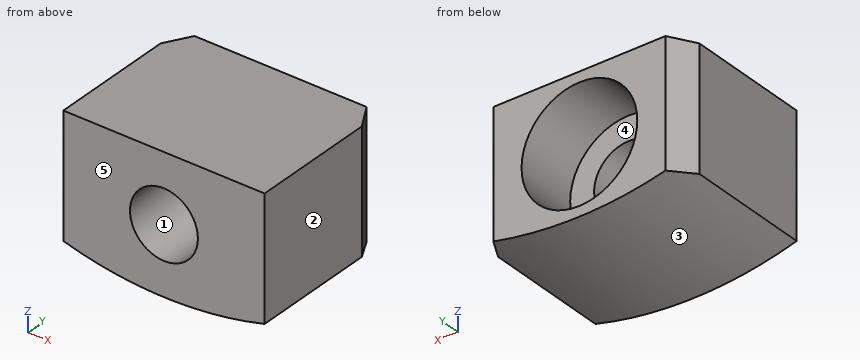
```python
from build123d import *
from OCP.BRepFilletAPI import BRepFilletAPI_MakeChamfer

# Parameters (mm, degrees)
SKETCH1_W                = 8
SKETCH1_H                = 5.7
EXTRUDED_BOSS_BASE_DEPTH = 3
LEGACY_HOLE_D            = 2.7
LEGACY_HOLE_CBORE_D      = 4.6
LEGACY_HOLE_CBORE_DEPTH  = 2.5
FILLET_2_SIZE            = 1
FILLET_2_SIZE2           = 0.577350269
SKETCH4_R                = 15.717506164
SKETCH4_R_2              = 14.9
EXTRUDED_CUT_DEPTH       = 8.810249676


with BuildPart() as part:
    # Sketch1 → Extruded Boss/Base (new, symmetric)
    with BuildSketch(Plane(origin=(0, 0, 0), x_dir=(1, 0, 0), z_dir=(0, 1, 0))):
        with Locations((0, 0.15)):
            Rectangle(SKETCH1_W, SKETCH1_H)
    extrude(amount=EXTRUDED_BOSS_BASE_DEPTH, both=True)

    # Legacy Hole (through all)
    with Locations(Plane(origin=(0, 3, 0), x_dir=(-1, 0, 0), z_dir=(0, 1, 0))):
        with Locations((0, 0)):
            CounterBoreHole(LEGACY_HOLE_D / 2, LEGACY_HOLE_CBORE_D / 2, LEGACY_HOLE_CBORE_DEPTH)

    # Fillet 2: one chamfer whose edges measure the first distance from different faces: ONE call of the kernel's chamfer builder (chamfer() names one face for all edges)
    fillet_2_edges_1 = [part.edges().sort_by_distance(p)[0] for p in [
        (4, 3, -0.15),
    ]]
    fillet_2_side_1 = [part.faces().sort_by_distance(p)[0] for p in [
        (4, 0, -0.15),
    ]]
    fillet_2_edges_2 = [part.edges().sort_by_distance(p)[0] for p in [
        (-4, 3, -0.15),
    ]]
    fillet_2_side_2 = [part.faces().sort_by_distance(p)[0] for p in [
        (-4, 0, -0.15),
    ]]
    fillet_2 = BRepFilletAPI_MakeChamfer(part.part.solid().wrapped)
    for e in fillet_2_edges_1:
        fillet_2.Add(FILLET_2_SIZE, FILLET_2_SIZE2, e.wrapped, fillet_2_side_1[0].wrapped)  # the first distance lies on this face
    for e in fillet_2_edges_2:
        fillet_2.Add(FILLET_2_SIZE, FILLET_2_SIZE2, e.wrapped, fillet_2_side_2[0].wrapped)  # the first distance lies on this face
    add(Compound.cast(fillet_2.Shape()), mode=Mode.REPLACE)

    # Sketch4 → Extruded Cut (cut, through all)
    with BuildSketch(Plane(origin=(0, 3, 0), x_dir=(1, 0, 0), z_dir=(0, 1, 0))):
        with Locations((0, -12.2)):
            Circle(SKETCH4_R)
        with Locations((0, -12.2)):
            Circle(SKETCH4_R_2, mode=Mode.SUBTRACT)
    extrude(amount=-EXTRUDED_CUT_DEPTH, mode=Mode.SUBTRACT)


solid = part.part
```
Could you check a few things on this model? Use its own coordinates, in mm. Face numbers are marked on the shaded views. A direction names the side the tool comes from. Coordinates: 2 decimals unless noted, no trailing zeros. Loops run counter-clockwise (first coordinate to the right, second up) from the corner with the lowest first, then second, coordinate; pieces in that order, holes last.
1) Imagine slicing it at D-D (z = 1.9). List the corners of the cut face in (x, y) for me.
Reported:
outline: (-4, -3) - (4, -3) - (4, 2) - (3.42, 3) - (1.3, 3) - (1.3, 0.5) - (-1.3, 0.5) - (-1.3, 3) - (-3.42, 3) - (-4, 2) - close
2) Imagine slicing it at A-A (z = 0). List the corners of the cut face in (x, y) for me.
Reported:
outline: (-4, -3) - (-1.35, -3) - (-1.35, 0.5) - (-2.3, 0.5) - (-2.3, 3) - (-3.42, 3) - (-4, 2) - close; (1.35, -3) - (4, -3) - (4, 2) - (3.42, 3) - (2.3, 3) - (2.3, 0.5) - (1.35, 0.5) - close
3) Imagine slicing it at C-C (y = -0.25). List the corners of the cut face in (x, z) for me, and give its area (3 significant figures).
Reported:
outline: (-4, -2.15) arc R14.9 ccw to (4, -2.15) - (4, 2.7) - (-4, 2.7) - close; hole circle Ø2.7 at (0, 0)
area: 36.0 mm2
4) Please list where these lines run through material, in increasing order: line 1 along Z through (x, y) = (0, 1.6); line 2 along Z through (x, y) = (0, -1.35); line 3 along Y through (x, z) = (1.75, 0.25).
Reported:
line 1: z = -2.7 to -2.3, 2.3 to 2.7
line 2: z = -2.7 to -1.35, 1.35 to 2.7
line 3: y = -3 to 0.5
5) Will these pins go through, and if not, where does the flat tip stop? pin 1 Ø1 at (x, y) = (1.5, 1) entering from -Z; pin 2 Ø3 at (x, z) = (1, 0.5) entering from -Y.
Reported:
pin 1: stops at z = -2.67
pin 2: stops at y = -3
6) Imagine slicing it at B-B (x = 0). List the corners of the cut face in (y, z) for me.
Reported:
outline: (-3, -2.7) - (3, -2.7) - (3, -2.3) - (0.5, -2.3) - (0.5, -1.35) - (-3, -1.35) - close; (-3, 1.35) - (0.5, 1.35) - (0.5, 2.3) - (3, 2.3) - (3, 2.7) - (-3, 2.7) - close
7) Thinking about a two-plate mould opening in Z: for the marked faces 1, 2 and 3, which applies, released by +Z, released by -Z, zero draft, split by the parting line, or undercut?
Reported:
face 1: undercut
face 2: zero draft
face 3: released by -Z
8) Which directions (+Z, -Z, +X, -X, +Y, -Y) give clear straight access to the entire face, cutting with the end or side of a thin tool? Please do the marked faces 4 and 5.
Reported:
face 4: +Y
face 5: +Z, -Z, +X, -X, -Y
